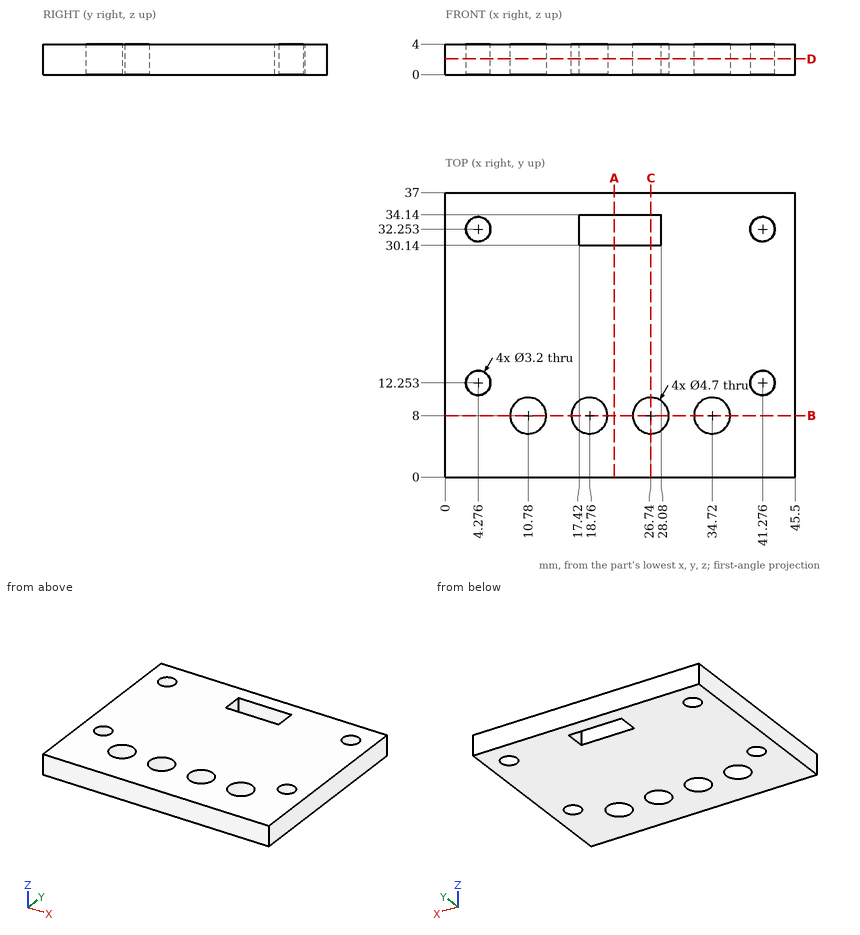
Could you check a few things on this drawing? It's one solid part, dimensions in mm from its lowest x, y, z. Give positions to 0.01 mm unless a question says otherwise; leave off trailing zeros. Order: outer loops, then holes, each group sorted by start corner. A loop starts at its lowest first (then second) coordinate and runs counter-clockwise, first axis right, second up. Notation, with made-up numbers: (60.25, 26) - (98.25, 26) arc R37 ccw to (98.25, 62) - close; hole circle Ø3 at (15.5, 34). An arc over 180 degrees is marked (long way). Answer as a JSON object with one key per item and string values. Group by question number.
Item 1: If we section it at D-D on z = 2.05: Give the number of separate pieces and of enclosed holes in the cut face, and give its area (3 significant figures).
Item 2: If we section it at C-C on x = 26.74: Please give me the cut outline in (y, z).
Item 3: If we section it at B-B on y = 8: Please give me the cut outline in (x, z), and give its area (3 significant figures).
Item 4: Please list where these lines run through material, in increasing order: probe 1 along Y at (x, z) = (26.5, 1.55); probe 2 along Y at (x, z) = (3.5, 0.4) (1 decimal); probe 3 along X at (y, z) = (34, 0.65).
Item 5: If we section it at A-A on x = 22: Please give me the cut outline in (y, z), and give its area (3 significant figures).
Result set:
{
 "1": {"separate pieces": "1", "enclosed holes": "9", "area": "1,540 mm²"},
 "2": {"outline": "(0, 0) - (5.65, 0) - (5.65, 4) - (0, 4) - close; (10.35, 0) - (30.14, 0) - (30.14, 4) - (10.35, 4) - close; (34.14, 0) - (37, 0) - (37, 4) - (34.14, 4) - close"},
 "3": {"outline": "(0, 0) - (8.43, 0) - (8.43, 4) - (0, 4) - close; (13.13, 0) - (16.41, 0) - (16.41, 4) - (13.13, 4) - close; (21.11, 0) - (24.39, 0) - (24.39, 4) - (21.11, 4) - close; (29.09, 0) - (32.37, 0) - (32.37, 4) - (29.09, 4) - close; (37.07, 0) - (45.5, 0) - (45.5, 4) - (37.07, 4) - close", "area": "107 mm²"},
 "4": {"probe 1": "0 to 5.66, 10.34 to 30.14, 34.14 to 37", "probe 2": "0 to 10.9, 13.7 to 30.9, 33.7 to 37", "probe 3": "0 to 17.42, 28.08 to 45.5"},
 "5": {"outline": "(0, 0) - (30.14, 0) - (30.14, 4) - (0, 4) - close; (34.14, 0) - (37, 0) - (37, 4) - (34.14, 4) - close", "area": "132 mm²"}
}
